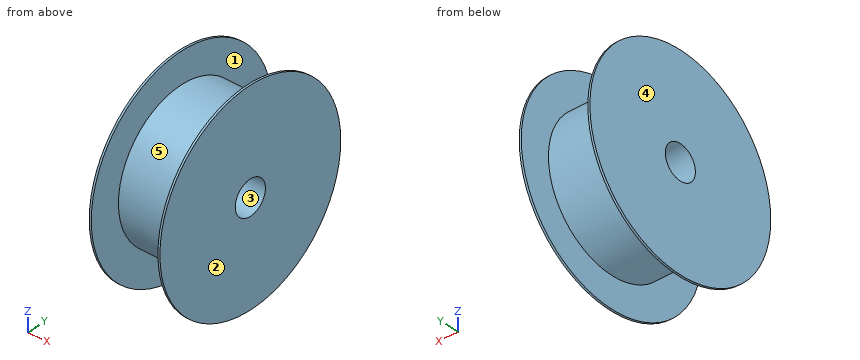
Autodesk Inventor part; units mm, degrees
ref_plane "YZ Plane" through (0, 0, 0) normal (1, 0, 0) x (0, 1, 0)
ref_plane "XZ Plane" through (0, 0, 0) normal (0, 1, 0) x (-1, 0, 0)
ref_plane "XY Plane" through (0, 0, 0) normal (0, 0, 1) x (1, 0, 0)
sketch "Sketch1" plane through (0, 0, 0) normal (0, 0, 1) x (1, 0, 0)
  line L0 (0, 0) -> (52, 0)
  line L1 (52, 0) -> (52, 150)
  line L2 (52, 150) -> (49, 150)
  line L3 (49, 150) -> (49, 105)
  line L4 (49, 105) -> (0, 105)
  line L5 (0, 105) -> (0, 0)
  line L6 (0, 25) -> (52, 25)
  dimension "d0" = 52
  dimension "d1" = 150
  dimension "d2" = 3
  dimension "d3" = 25
  dimension "d4" = 105
revolve "Revolution1" add sketch "Sketch1" angle 360 about axis through (0, 0, 0) along (1, 0, 0) contours L5 L4 L3 L2 L1 L6
mirror "Mirror1" about plane through (0, 65, 0) normal (-1, 0, 0) of "Revolution1"
properties part number "rolka_filamentu"
The model under review builds one solid part; all positions refer to its coordinate system, in mm. Face numbers are marked on the shaded views. A direction names the side the tool comes from. Give positions to 0.01 mm unless a question says otherwise; leave off trailing zeros. Order: outer loops, then holes, each group sorted by start corner. A loop starts at its lowest first (then second) coordinate and runs counter-clockwise, first axis right, second up. Notation, with made-up numbers: M 54.25,33 L 76.25,33 A29 ccw 76.25,57 Z; hole C 55,14 d5. An arc over 180 degrees is marked long. Use one line per item in the form item = value. Start each with the question number.
Item 1: We need section D-D on y = -57. Give the boundary of the cut face in (x, z), plus the area to 3 significant figures.
Item 2: We need section C-C on x = -41. Give the boundary of the cut face in (y, z), plus the area to 3 significant figures.
Item 3: For the marked faces 1 and 2, list the 3-axis set-ups (+Z, -Z, +X, -X, +Y, -Y) from which the entire face can be reached by the end or side of a thin tool; tool diameter is ignored.
Item 4: The part is to be moulded in two halves that separate along Z. For the marked faces 3, 4 and 5, say which applies: pulls with the +Z half, pulls with the -Z half, needs draft (parallel to the pull), parting line crosses it, or undercut.
Item 5: We need section A-A on y = 0. Give the boundary of the cut face in (x, z).
Item 6: Insertion check: pin 1 Ø3 at (x, z) = (20, 79) entering from +Y; pin 2 Ø10 at (x, z) = (-12.5, -87.5) entering from +Y; pin 3 Ø10 at (x, y) = (-3, -39.5) entering from +Z. Each pin has a flat end and moves straight along its axis. Give the tip position at first contact, or say it passes through.
Item 7: To check wall thickness, follow line 1 along X through (y, z) = (130, -24); line 2 along Z through (x, y) = (9, 0); line 3 along Z through (x, y) = (26, -6.5). State the ranges of each line that lie inside material, in increasing order. Write a range as from..to.
Completed:
q1.outline = M -52,-138.75 L -49,-138.75 L -49,-88.18 L 49,-88.18 L 49,-138.75 L 52,-138.75 L 52,138.75 L 49,138.75 L 49,88.18 L -49,88.18 L -49,138.75 L -52,138.75 Z
q1.area = 18,900 mm²
q2.outline = C 0,0 d210; hole C 0,0 d50
q2.area = 32,700 mm²
q3.face_1 = none
q3.face_2 = +Z, -Z, +X, +Y, -Y
q4.face_3 = undercut
q4.face_4 = needs draft
q4.face_5 = parting line crosses it
q5.outline = M -52,-150 L -49,-150 L -49,-105 L 49,-105 L 49,-150 L 52,-150 L 52,-25 L -52,-25 Z; M -52,25 L 52,25 L 52,150 L 49,150 L 49,105 L -49,105 L -49,150 L -52,150 Z
q6.pin_1 = 70.84
q6.pin_2 = 64.95
q6.pin_3 = 99.17
q7.line_1 = -52..-49, 49..52
q7.line_2 = -105..-25, 25..105
q7.line_3 = -104.8..-24.14, 24.14..104.8
